Here's how the part is built. I have some questions about the finished solid (model axes, mm). Coordinates: 2 decimals unless noted, no trailing zeros. Write each loop counter-clockwise with the first axis right and the second up, starting at its lowest first coordinate (ties: lowest second). Pieces come first, ordered by that corner, then holes. Notation, with made-up numbers: M 83,62 L 139,62 A12 ccw 139,69 Z; hole C 16,75 d9. An arc over 180 degrees is marked long. Use a Markdown table: item, result.
```python
from build123d import *

# Parameters (mm, degrees)
F0_R     = 12.7
F0_R_2   = 44.45
F1_DEPTH = 6.35


# Not quite as in the source:
# - a length typed as a fraction of an inch, garbled in the dataset ("3 / 203.2 mm" for 3/8 in), is restored


with BuildPart() as f1:
    # F0 (on Front) → F1 (new body)
    with BuildSketch(Plane.XZ):
        with BuildLine():
            ThreePointArc((-75.1176136364, -31.7315448688), (-59.3475236203, -34.5646316236), (-46.13671875, -43.6308741946))
            ThreePointArc((-46.13671875, -43.6308741946), (0, -63.5), (46.13671875, -43.6308741946))
            ThreePointArc((46.13671875, -43.6308741946), (59.3475236203, -34.5646316236), (75.1176136364, -31.7315448688))
            ThreePointArc((75.1176136364, -31.7315448688), (107.95, 0), (75.1176136364, 31.7315448688))
            ThreePointArc((75.1176136364, 31.7315448688), (59.3475236203, 34.5646316236), (46.13671875, 43.6308741946))
            ThreePointArc((46.13671875, 43.6308741946), (0.1332471885, 63.4998601982), (-45.9532044665, 43.8241143579))
            ThreePointArc((-45.9532044665, 43.8241143579), (-59.3485408179, 34.6632102418), (-75.3109250125, 31.7375494591))
            ThreePointArc((-75.3109250125, 31.7375494591), (-107.9498527345, -0.0967023051), (-75.1176136364, -31.7315448688))
        make_face()
        with Locations((-76.2, 0)):
            Circle(F0_R, mode=Mode.SUBTRACT)
        Circle(F0_R_2, mode=Mode.SUBTRACT)
        with Locations((76.2, 0)):
            Circle(F0_R, mode=Mode.SUBTRACT)
    extrude(amount=F1_DEPTH)


solid = f1.part
```
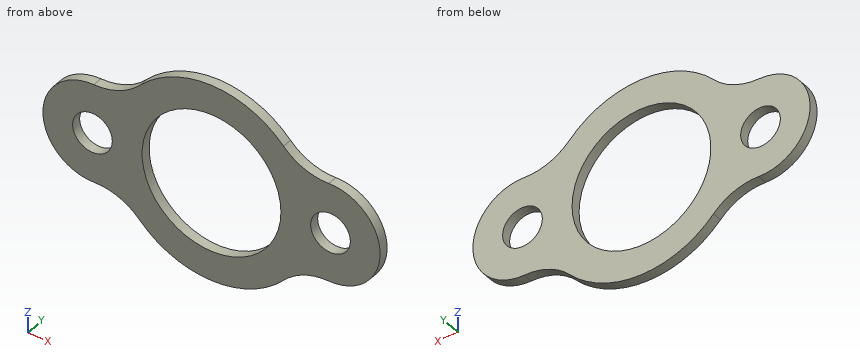
1. I need wall thicknesses on probe 1 along Z at (x, y) = (76.2, -3.5); probe 2 along X at (y, z) = (-3.5, 1); probe 3 along Z at (x, y) = (0, -5). Which ranges of each line are inside material? Lowest first, please.
Answers follow:
| item | result |
|---|---|
| probe 1 | z = -31.75 to -12.7, 12.7 to 31.75 |
| probe 2 | x = -107.93 to -88.86, -63.54 to -44.44, 44.44 to 63.54, 88.86 to 107.93 |
| probe 3 | z = -63.5 to -44.45, 44.45 to 63.5 |
2. Suppose I cut it at A-A on x = 0. Write out the boundary of the cut face in (y, z).
Answers follow:
| item | result |
|---|---|
| outline | M -6.35,-63.5 L 0,-63.5 L 0,-44.45 L -6.35,-44.45 Z; M -6.35,44.45 L 0,44.45 L 0,63.5 L -6.35,63.5 Z |
3. Suppose I cut it at B-B on z = 0. Write out the boundary of the cut face in (x, y), and give its area (3 significant figures).
Answers follow:
| item | result |
|---|---|
| outline | M -107.95,-6.35 L -88.9,-6.35 L -88.9,0 L -107.95,0 Z; M -63.5,-6.35 L -44.45,-6.35 L -44.45,0 L -63.5,0 Z; M 44.45,-6.35 L 63.5,-6.35 L 63.5,0 L 44.45,0 Z; M 88.9,-6.35 L 107.95,-6.35 L 107.95,0 L 88.9,0 Z |
| area | 484 mm2 |
4. Will these pins go through, and if not, where does the flat tip stop? pin 1 Ø3 at (x, y) = (77, -5.5) entering from +Z; pin 2 Ø3 at (y, z) = (-0.5, 41.5) entering from -X; pin 3 Ø2 at (y, z) = (-1, -45.5) entering from -X.
Answers follow:
| item | result |
|---|---|
| pin 1 | stops at z = 31.75 |
| pin 2 | stops at x = -50.17 |
| pin 3 | stops at x = -45.3 |
5. Suppose I cut it at C-C on y = -4. Write out the boundary of the cut face in (x, z).
Answers follow:
| item | result |
|---|---|
| outline | M -75.31,31.74 A31.75 ccw long -75.12,-31.73 A38.1 cw -46.14,-43.63 A63.5 ccw 46.14,-43.63 A38.1 cw 75.12,-31.73 A31.75 ccw long 75.12,31.73 A38.1 cw 46.14,43.63 A63.5 ccw -45.95,43.82 A39.06 cw Z; hole C -76.2,0 d25.4; hole C 0,0 d88.9; hole C 76.2,0 d25.4 |
6. Suppose I cut it at D-D on z = -40. Write out the boundary of the cut face in (x, y), and give its area (3 significant figures).
Answers follow:
| item | result |
|---|---|
| outline | M -50.09,-6.35 L -19.39,-6.35 L -19.39,0 L -50.09,0 Z; M 19.39,-6.35 L 50.09,-6.35 L 50.09,0 L 19.39,0 Z |
| area | 390 mm2 |
